Work out the finished part from the listing and answer in its coordinate system (mm). A direction names the side the tool comes from. Give positions to 0.01 mm unless a question says otherwise; leave off trailing zeros. Loops run counter-clockwise (first coordinate to the right, second up) from the corner with the lowest first, then second, coordinate; pieces in that order, holes last. Notation, with made-up numbers: (71.5, 30.5) - (107.5, 30.5) arc R25 ccw to (107.5, 45.5) - close; hole circle Ø8 at (-12, 6.25). An arc over 180 degrees is marked (long way). One line per question, with ' | ' between items. Start each with the question number.
1. Each of these flat-tipped pins is pushed along its axis until it touches: pin 1 (1 mm diameter, centred on x = 14.5, y = 1.5, fed in from -Z); pin 2 (1 mm diameter, centred on y = 2.5, z = 2, fed in from -X); pin 3 (1 mm diameter, centred on y = 3, z = -2.5, fed in from +X). Where does it stop, or does it pass through?
2. For a pull along Z with two mould halves and no side action, classify faces 1 (the face through (-17.907, 2, 11)), 2 (the face through (-24, 2, 12.192)), 3 (the face through (-26.67, 2, 0)) as released by +Z, released by -Z, zero draft, split by the parting line, or undercut.
3. Section D-D (z = 0.75) is taken. Determine the outline of the cut face in (x, y) (3 decimals).
4. Find the intervals of material crossed by line 1 (X direction, y = 2.05, z = -10) (3 decimals); line 2 (Z direction, x = 27, y = 2.55); line 3 (X direction, y = 0.35, z = 1.5), in increasing order.
5. Which of the six approach directions +Z, -Z, +X, -X, +Y, -Y give full straight-line access (tool end or side, diameter ignored) to faces 4 (the face through (26.67, 2, 0)), 5 (the face through (12, 2, 9.017)), 6 (the face through (12, 2, -9.017))?
6. Section C-C (x = 7) is taken. Determine the outline of the cut face in (y, z) (3 decimals).
7. Section B-B (y = 1.35) is taken. Determine the outline of the cut face in (x, z) (3 decimals), plus the area to 3 significant figures.
8. Section A-A (z = 10.5) is taken. Determine the outline of the cut face in (x, y) (3 decimals).
from build123d import *

# Parameters (mm, degrees)
SKETCH1_W           = 59.69
SKETCH1_H           = 24.384
BOSS_EXTRUDE2_DEPTH = 3.175
SKETCH3_W           = 11.938
SKETCH3_H           = 3.175
CUT_EXTRUDE2_DEPTH  = 3.175
LPATTERN2_COUNT     = 2
LPATTERN2_PITCH     = 23.876
SKETCH4_W           = 6.35
SKETCH4_H           = 8.128
CUT_EXTRUDE3_DEPTH  = 3.175


with BuildPart() as part:
    # Sketch1 → Boss-Extrude2 (new body)
    with BuildSketch(Plane(origin=(0, 0, 0), x_dir=(1, 0, 0), z_dir=(0, 1, 0))):
        Rectangle(SKETCH1_W, SKETCH1_H)
    extrude(amount=BOSS_EXTRUDE2_DEPTH)

    # Sketch3 → Cut-Extrude2 (cut)
    with BuildSketch(Plane(origin=(0, 3.175, 0), x_dir=(1, 0, 0), z_dir=(0, 1, 0))):
        with Locations((11.938, 10.6045)):
            Rectangle(SKETCH3_W, SKETCH3_H)
        with Locations((11.938, -10.6045)):
            Rectangle(SKETCH3_W, SKETCH3_H)
    cut_extrude2 = extrude(amount=-CUT_EXTRUDE2_DEPTH, mode=Mode.SUBTRACT)

    # LPattern2: Cut-Extrude2 ×2
    with Locations(*[(-i * LPATTERN2_PITCH, 0, 0) for i in range(1, LPATTERN2_COUNT)]):
        add(cut_extrude2, mode=Mode.SUBTRACT)

    # Sketch4 → Cut-Extrude3 (cut)
    with BuildSketch(Plane(origin=(0, 3.175, 0), x_dir=(1, 0, 0), z_dir=(0, 1, 0))):
        with Locations((-29.845, 0)):
            Rectangle(SKETCH4_W, SKETCH4_H)
        with Locations((29.845, 0)):
            Rectangle(SKETCH4_W, SKETCH4_H)
    extrude(amount=-CUT_EXTRUDE3_DEPTH, mode=Mode.SUBTRACT)


solid = part.part
Conclusion:
1) pin 1: z = -9.02 | pin 2: x = -26.67 | pin 3: x = 26.67
2) face 1: zero draft | face 2: released by +Z | face 3: undercut
3) outline: (-26.67, 0) - (26.67, 0) - (26.67, 3.175) - (-26.67, 3.175) - close
4) line 1: -29.845 to -17.907, -5.969 to 5.969, 17.907 to 29.845 | line 2: -12.19 to -4.06, 4.06 to 12.19 | line 3: -26.67 to 26.67
5) face 4: +X, +Y, -Y | face 5: +Z, +Y, -Y | face 6: -Z, +Y, -Y
6) outline: (0, -9.017) - (3.175, -9.017) - (3.175, 9.017) - (0, 9.017) - close
7) outline: (-29.845, -12.192) - (-17.907, -12.192) - (-17.907, -9.017) - (-5.969, -9.017) - (-5.969, -12.192) - (5.969, -12.192) - (5.969, -9.017) - (17.907, -9.017) - (17.907, -12.192) - (29.845, -12.192) - (29.845, -4.064) - (26.67, -4.064) - (26.67, 4.064) - (29.845, 4.064) - (29.845, 12.192) - (17.907, 12.192) - (17.907, 9.017) - (5.969, 9.017) - (5.969, 12.192) - (-5.969, 12.192) - (-5.969, 9.017) - (-17.907, 9.017) - (-17.907, 12.192) - (-29.845, 12.192) - (-29.845, 4.064) - (-26.67, 4.064) - (-26.67, -4.064) - (-29.845, -4.064) - close | area: 1,250 mm²
8) outline: (-29.845, 0) - (-17.907, 0) - (-17.907, 3.175) - (-29.845, 3.175) - close; (-5.969, 0) - (5.969, 0) - (5.969, 3.175) - (-5.969, 3.175) - close; (17.907, 0) - (29.845, 0) - (29.845, 3.175) - (17.907, 3.175) - close
